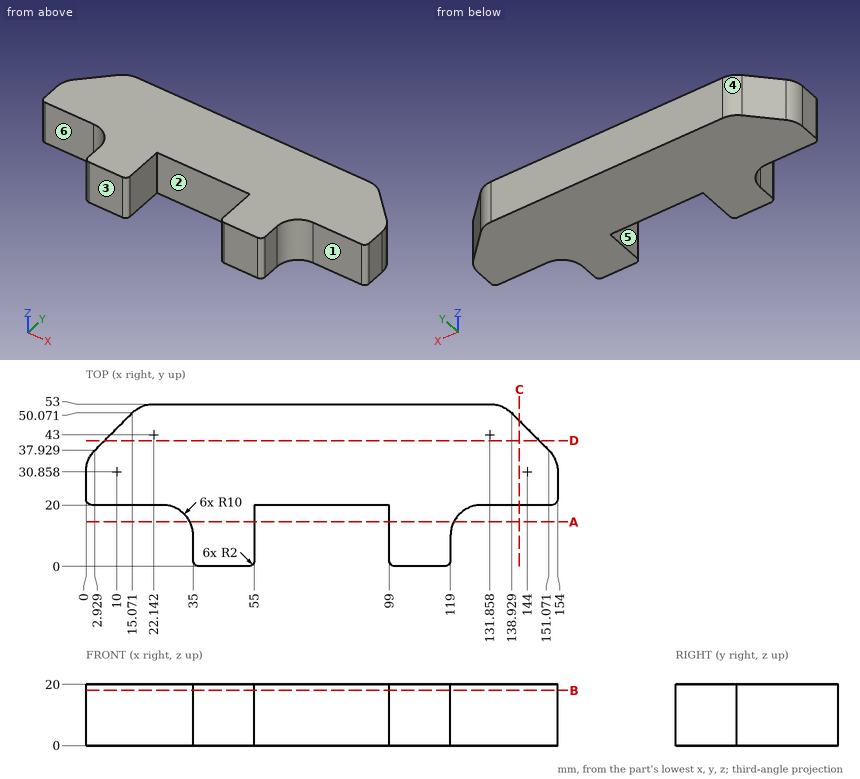
Can you work these out from the drawing? Everything is in mm from the part's minimum corner. A direction names the side the tool comes from. Give positions to 0.01 mm unless a question says otherwise; leave off trailing zeros. Order: outer loops, then holes, each group sorted by start corner. A loop starts at its lowest first (then second) coordinate and runs counter-clockwise, first axis right, second up.
1. We'd pull the mould along X, two halves only. Please class the marked faces 4, 5 and 6: pulls with the +X half, pulls with the -X half, needs draft (parallel to the pull), parting line crosses it, or undercut.
2. Suppose I cut it at B-B (z = 18). List the corners of the cut face in (x, y) for me, plus the area to 3 significant figures.
3. For the marked faces 1, 2 and 3, which set-ups out of +Z, -Z, +X, -X, +Y, -Y let a thin tool reach every point of the face, with its end or its side?
4. I need wall thicknesses on L1, parallel to X at y = 2, z = 13.75; L2, parallel to X at y = 31, z = 14.5; L3, parallel to Y at x = 73, z = 5.5. Which ranges of each line are inside material? Lowest first, please.
5. Suppose I cut it at D-D (y = 41). List the corners of the cut face in (x, z) for me, plus the area to 3 significant figures.
6. Suppose I cut it at C-C (x = 141.5). List the corners of the cut face in (y, z) for me.
7. Will these pins go through, and if not, where does the flat tip stop? P1, Ø10, axis at y = 6.5, z = 15, coming from the +X side; P2, Ø6.5, axis at y = 7, z = 8, coming from the +X side; P3, Ø4, axis at x = 122, z = 11.5, coming from the -Y side.
8. Suppose I cut it at A-A (y = 14.5). List the corners of the cut face in (x, z) for me.
Solved:
1. face 4: pulls with the -X half
1. face 5: undercut
1. face 6: needs draft
2. outline: (0, 22) arc R2 ccw to (2, 20) - (25, 20) arc R10 cw to (35, 10) - (35, 2) arc R2 ccw to (37, 0) - (53, 0) arc R2 ccw to (55, 2) - (55, 20) - (99, 20) - (99, 2) arc R2 ccw to (101, 0) - (117, 0) arc R2 ccw to (119, 2) - (119, 10) arc R10 cw to (129, 20) - (152, 20) arc R2 ccw to (154, 22) - (154, 30.86) arc R10 ccw to (151.07, 37.93) - (138.93, 50.07) arc R10 ccw to (131.86, 53) - (22.14, 53) arc R10 ccw to (15.07, 50.07) - (2.93, 37.93) arc R10 ccw to (0, 30.86) - close
2. area: 5,590 mm2
3. face 1: +Z, -Z, +X, -Y
3. face 2: +Z, -Z, -Y
3. face 3: +Z, -Z, +X, -X, -Y
4. L1: x = 35 to 55, 99 to 119
4. L2: x = 0 to 154
4. L3: y = 20 to 53
5. outline: (6, 0) - (148, 0) - (148, 20) - (6, 20) - close
5. area: 2,840 mm2
6. outline: (20, 0) - (47.5, 0) - (47.5, 20) - (20, 20) - close
7. P1: stops at x = 119.11
7. P2: stops at x = 119
7. P3: stops at y = 14.36
8. outline: (33.93, 0) - (55, 0) - (55, 20) - (33.93, 20) - close; (99, 0) - (120.07, 0) - (120.07, 20) - (99, 20) - close
